from build123d import *

# Parameters (mm, degrees)
SKETCH_1_R               = 12
EXTRUDE_1_DEPTH          = 31
HOLE_WIZARD_M10_1_D      = 8.5
CHAMFER_1_SIZE           = 1
CUT_EXTRUDE_1_DEPTH      = 36.341194094
CUT_EXTRUDE_1_DEPTH_BACK = 36.341194094
SKETCH_5_R               = 31


with BuildPart() as part:
    # 草图1 → 凸台-拉伸1 (new body)
    with BuildSketch(Plane(origin=(0, 0, 0), x_dir=(1, 0, 0), z_dir=(0, 1, 0))):
        with Locations(Location((0, 0, 0), (0, 0, 270))):
            Circle(SKETCH_1_R)
    extrude(amount=EXTRUDE_1_DEPTH)

    # M10 螺纹孔1 (through all)
    with Locations(Plane(origin=(0, 31, 0), x_dir=(1, 0, 0), z_dir=(0, 1, 0))):
        with Locations((0, 0)):
            Hole(HOLE_WIZARD_M10_1_D / 2)

    # 倒角1
    chamfer_1_edges = [part.edges().sort_by_distance(p)[0] for p in [
        (0, 0, -12),
        (0, 31, -12),
    ]]
    chamfer(chamfer_1_edges, length=CHAMFER_1_SIZE)

    # 草图5 → 切除-拉伸1 (cut, two sides: drawn at the far end of the back side and taken through both)
    with BuildSketch(Plane.XY.offset(-CUT_EXTRUDE_1_DEPTH_BACK)):
        with Locations((-40, 35)):
            Circle(SKETCH_5_R)
    extrude(amount=CUT_EXTRUDE_1_DEPTH + CUT_EXTRUDE_1_DEPTH_BACK, mode=Mode.SUBTRACT)


solid = part.part
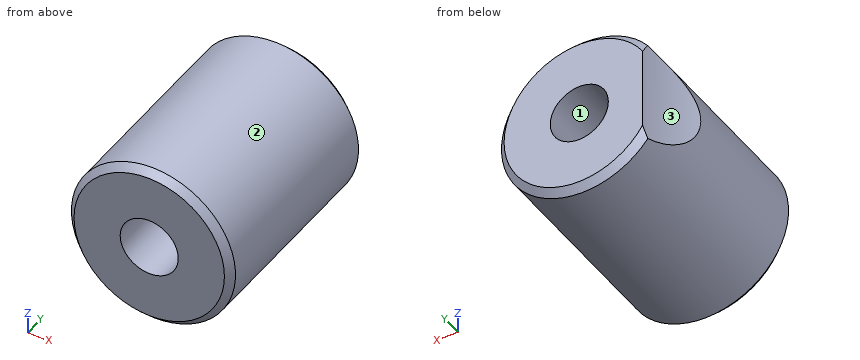
Geometry check sheet. Reference: the model listing, model coordinates, mm. Face numbers are marked on the shaded views. Coordinates: 2 decimals unless noted, no trailing zeros. Write each loop counter-clockwise with the first axis right and the second up, starting at its lowest first coordinate (ties: lowest second). Pieces come first, ordered by that corner, then holes. Notation, with made-up numbers: (-18, 28) -> (32, 28) arc R21 ccw to (32, 67) -> close; hole circle Ø2 at (59, -29.5). An arc over 180 degrees is marked (long way). One line per question, with ' | ' between items.
1. Draft check along Z on the marked faces 1, 2 and 3. Enter one of: +Z half, -Z half, draft (parallel to the pull), parting line (faces both ways), or undercut.
Answers:
face 1: undercut | face 2: parting line | face 3: draft
2. Cross-section at C-C on y = 4.5. Record the cut outline in (x, z), and give its area (3 significant figures).
Answers:
outline: circle Ø24 at (0, 0); hole circle Ø8.5 at (0, 0) | area: 396 mm²
3. Cross-section at B-B on x = 0. Record the cut outline in (y, z).
Answers:
outline: (0, -11) -> (1, -12) -> (30, -12) -> (31, -11) -> (31, -4.25) -> (0, -4.25) -> close; (0, 4.25) -> (31, 4.25) -> (31, 11) -> (30, 12) -> (1, 12) -> (0, 11) -> close
4. Thickness scan on probe 1 along Z at (x, y) = (0, 25); probe 2 along Z at (x, y) = (-1.5, 10); probe 3 along X at (y, z) = (22.5, 0.75). Record the ranges inside material, lowest first. Write a range as from..to.
Answers:
probe 1: z = -12..-4.25, 4.25..12 | probe 2: z = -11.91..-3.98, 3.98..11.91 | probe 3: x = -11.63..-4.18, 4.18..11.98
5. Depth check by flat-ended pin: pin 1 Ø10 at (y, z) = (5, 5) entering from +X; pin 2 Ø3 at (x, y) = (-2.5, 9) entering from +Z; pin 3 Ø1.5 at (x, y) = (-3, 4.5) entering from -Z; pin 4 Ø8 at (y, z) = (10.5, -7.5) entering from +X. Enter the tip coordinate at first touch or a pass-through.
Answers:
pin 1: stops at x = 12 | pin 2: stops at z = 11.96 | pin 3: stops at z = -11.79 | pin 4: stops at x = 11.48
6. Cross-section at A-A on z = 0. Record the cut outline in (x, y), and give its area (3 significant figures).
Answers:
outline: (-12, 1) -> (-11, 0) -> (-4.25, 0) -> (-4.25, 31) -> (-9.26, 31) arc R31 cw to (-12, 21.7) -> close; (4.25, 0) -> (11, 0) -> (12, 1) -> (12, 30) -> (11, 31) -> (4.25, 31) -> close | area: 464 mm²
